Read the model definition and answer for the solid it produces. Units are mm, in the model's axes. A direction names the side the tool comes from. Give positions to 0.01 mm unless a question says otherwise; leave off trailing zeros. Write each loop counter-clockwise with the first axis right and the second up, starting at its lowest first coordinate (ties: lowest second). Pieces come first, ordered by that corner, then holes. Notation, with made-up numbers: (0, 4.5) -> (30, 4.5) arc R15 ccw to (30, 17.5) -> close; hole circle Ø3 at (-2.75, 79.25). An arc over 180 degrees is marked (long way). Use a Markdown table: item, result.
from build123d import *

# Parameters (mm, degrees)
SKETCH1_R           = 7.75
SKETCH1_W           = 44
SKETCH1_H           = 24
BOSS_EXTRUDE1_DEPTH = 65
SKETCH5_W           = 65
SKETCH5_H           = 15
SKETCH5_R           = 4.05
BOSS_EXTRUDE4_DEPTH = 83
CHAMFER1_SIZE       = 10
SKETCH6_R           = 2.75
CUT_EXTRUDE1_DEPTH  = 15
SKETCH8_R           = 2.75
BOSS_EXTRUDE5_DEPTH = 3
EXTRUDE_THIN2_DEPTH = 20
CHAMFER2_SIZE       = 5
CHAMFER3_SIZE       = 5


with BuildPart() as part:
    # Sketch1 → Boss-Extrude1 (new body)
    with BuildSketch(Plane.XY):
        Polygon((31.75, 17), (-31.75, 17), (-41.5, 17), (-41.5, -17), (-31.75, -17), (31.75, -17), (41.5, -17), (41.5, 17), align=None)
        with Locations((-31.75, 0)):
            Circle(SKETCH1_R, mode=Mode.SUBTRACT)
        with Locations((31.75, 0)):
            Circle(SKETCH1_R, mode=Mode.SUBTRACT)
        Rectangle(SKETCH1_W, SKETCH1_H, mode=Mode.SUBTRACT)
    extrude(amount=BOSS_EXTRUDE1_DEPTH)

    # Sketch5 → Boss-Extrude4 (add)
    with BuildSketch(Plane(origin=(41.5, 0, 0), x_dir=(0, 0, -1), z_dir=(1, 0, 0))):
        with Locations((-32.5, -24.5)):
            Rectangle(SKETCH5_W, SKETCH5_H)
        with Locations((-55, -24.5)):
            Circle(SKETCH5_R, mode=Mode.SUBTRACT)
        with Locations((-10, -24.5)):
            Circle(SKETCH5_R, mode=Mode.SUBTRACT)
    extrude(amount=-BOSS_EXTRUDE4_DEPTH)

    # Chamfer1
    chamfer1_edges = [part.edges().sort_by_distance(p)[0] for p in [
        (41.5, 17, 32.5),
    ]]
    chamfer(chamfer1_edges, length=CHAMFER1_SIZE)

    # Sketch6 → Cut-Extrude1 (cut)
    with BuildSketch(Plane(origin=(0, 12, 0), x_dir=(-1, 0, 0), z_dir=(0, -1, 0))):
        with Locations(Location((12, -32.5, 0), (0, 0, 90))):
            Circle(SKETCH6_R)
    extrude(amount=-CUT_EXTRUDE1_DEPTH, mode=Mode.SUBTRACT)



with BuildPart() as body_2:
    # Sketch8 → Boss-Extrude5 (new body)
    with BuildSketch(Plane(origin=(0, 37, 0), x_dir=(1, 0, 0), z_dir=(0, 1, 0))):
        Polygon((-41.5, -10), (-21, -32.5), (-41.5, -55), (-41.5, -65), (-31.5, -65), (-12, -41.5), (21.5, -65), (31.5, -65), (31.5, -55), (-3, -32.5), (31.5, -10), (31.5, 0), (21.5, 0), (-12, -21.847826087), (-31.5, 0), (-41.5, 0), align=None)
        with Locations(Location((-12, -32.5, 0), (0, 0, 90))):
            Circle(SKETCH8_R, mode=Mode.SUBTRACT)
    extrude(amount=BOSS_EXTRUDE5_DEPTH)


with BuildPart() as part_1:
    add(part.part)

    add(body_2.part)  # Extrude-Thin2 merges body 2
    # Sketch9 → Extrude-Thin2 (add)
    with BuildSketch(Plane(origin=(0, 37, 0), x_dir=(-1, 0, 0), z_dir=(0, -1, 0))):
        Polygon((41.5, -10), (41.5, 0), (31.5, 0), (31.5, -3), (38.5, -3), (38.5, -10), align=None)
        Polygon((-21.5, 0), (-31.5, 0), (-31.5, -10), (-28.5, -10), (-28.5, -3), (-21.5, -3), align=None)
    extrude_thin2 = extrude(amount=EXTRUDE_THIN2_DEPTH)

    # Mirror1: Extrude-Thin2 across plane
    add(extrude_thin2.mirror(Plane.XY.offset(32.5)))

    # Chamfer2
    chamfer2_edges = [part_1.edges().sort_by_distance(p)[0] for p in [
        (25, 37, 3),
        (28.5, 37, 6.5),
        (-38.5, 37, 58.5),
        (-35, 37, 62),
        (25, 37, 62),
        (28.5, 37, 58.5),
        (-38.5, 37, 6.5),
        (-35, 37, 3),
    ]]
    chamfer(chamfer2_edges, length=CHAMFER2_SIZE)

    # Chamfer3
    # the kernel refuses this chamfer: 5 mm, written as the material it takes off along each edge
    with BuildSketch(Plane(origin=(-41.5, 40, 42.14158506), x_dir=(0.9996219169112968, 0.0274958766105877, 0), z_dir=(0, 0, 1)), Plane(origin=(-54.35841494, 40, 65), x_dir=(0, 0.027495876610586317, -0.9996219169112968), z_dir=(1, 0, 0)), Plane(origin=(8.64158506, 40, 65), x_dir=(0, 0.027495876610586317, -0.9996219169112968), z_dir=(1, 0, 0)), Plane(origin=(31.5, 40, 77.85841494), x_dir=(-0.9996219169112968, 0.027495876610584936, 0), z_dir=(0, 0, -1)), Plane(origin=(44.35841494, 40, 0), x_dir=(0, 0.027495876610586317, 0.9996219169112968), z_dir=(-1, 0, 0)), Plane(origin=(-18.64158506, 40, 0), x_dir=(-1.1764219776297879e-15, 0.027495876610586317, 0.9996219169112968), z_dir=(-1, 0, 0)), Plane(origin=(-41.5, 40, -12.85841494), x_dir=(0.9996219169112968, 0.0274958766105877, 1.4205481831358163e-15), z_dir=(0, 0, 1))) as chamfer3_piece_1:
        Polygon((CHAMFER3_SIZE * 0.999621916911, -CHAMFER3_SIZE * 0.0274958766106), (-CHAMFER3_SIZE * 0.0274958766106, -CHAMFER3_SIZE * 0.999621916911), (0, 0), align=None)
    extrude(amount=35.71682988, mode=Mode.SUBTRACT)
    with BuildSketch(Plane(origin=(31.5, 40, 22.85841494), x_dir=(0.02749587661058701, -0.9996219169112968, 0), z_dir=(0, 0, -1))) as chamfer3_piece_2:
        Polygon((CHAMFER3_SIZE * 0.999621916911, CHAMFER3_SIZE * 0.0274958766106), (-CHAMFER3_SIZE * 0.0274958766106, CHAMFER3_SIZE * 0.999621916911), (0, 0), align=None)
    extrude(amount=35.71682988, mode=Mode.SUBTRACT)


solid = part_1.part
Item 1: A cutting plane is placed at D-D (x = -18). Give the vertices of the cut face in (y, z).
Return value:
| item | result |
|---|---|
| outline | (-32, 0) -> (-12, 0) -> (-12, 65) -> (-32, 65) -> close; (12, 0) -> (17, 0) -> (17, 65) -> (12, 65) -> close; (37, 15.13) -> (40, 15.13) -> (40, 48.73) -> (37, 48.73) -> close; hole circle Ø8.1 at (-24.5, 10); hole circle Ø8.1 at (-24.5, 55) |
Item 2: This flat-tipped pin is pushed along its axis until it touches: P1, Ø5, axis at y = 28.5, z = 6.5, coming from the +X side. Where does it stop, or does it pass through?
Return value:
| item | result |
|---|---|
| P1 | x = 31.5 |
Item 3: A cutting plane is placed at A-A (y = -10). Give the vertices of the cut face in (x, z).
Return value:
| item | result |
|---|---|
| outline | (-41.5, 0) -> (-22, 0) -> (-22, 65) -> (-41.5, 65) -> close; (22, 0) -> (41.5, 0) -> (41.5, 65) -> (22, 65) -> close |
Item 4: For a pull along Z with two mould halves and no side action, classify faces 1 (the face through (29, 29, 55)), 2 (the face through (31.5, 26, 60)), 3 (the face through (-39, 29, 55)) as +Z half, -Z half, draft (parallel to the pull), parting line (faces both ways), or undercut.
Return value:
| item | result |
|---|---|
| face 1 | undercut |
| face 2 | draft |
| face 3 | undercut |
Item 5: A tool of negligible diameter and unlimited length cuts with its end or side. For faces 4 (the face through (28.5, 25, 7)), 5 (the face through (-30.12, 38.48, 42.51)), 6 (the face through (22, 0, 32)), 7 (the face through (29, 29, 10)), from which of +Z, -Z, +X, -X, +Y, -Y can it reach the whole face along a straight path? Write none if from no direction.
Return value:
| item | result |
|---|---|
| face 4 | none |
| face 5 | -X, +Y |
| face 6 | +Z, -Z |
| face 7 | +X, -X |
Item 6: A cutting plane is placed at B-B (x = 35). Give the vertices of the cut face in (y, z).
Return value:
| item | result |
|---|---|
| outline | (-32, 0) -> (-7.04, 0) -> (-7.04, 65) -> (-32, 65) -> close; (7.04, 0) -> (13.5, 0) -> (13.5, 65) -> (7.04, 65) -> close; hole circle Ø8.1 at (-24.5, 10); hole circle Ø8.1 at (-24.5, 55) |
Item 7: Straight lines are drawn through the part: line 1 along Y through (x, z) = (-4, 42); line 2 along Y through (x, z) = (6.5, 10); line 3 along X through (y, z) = (28, 58). For each, find the intervals that lie inside material, in ascending order. Write a range as [from, to].
Return value:
| item | result |
|---|---|
| line 1 | [-32, -12], [12, 17], [37, 40] |
| line 2 | [-32, -28.55], [-20.45, -12], [12, 17], [37, 40] |
| line 3 | [-41.5, -38.5], [28.5, 31.5] |
Item 8: A cutting plane is placed at C-C (y = 21). Give the vertices of the cut face in (x, z), then the cut area to 3 significant figures.
Return value:
| item | result |
|---|---|
| outline | (-41.5, 0) -> (-31.5, 0) -> (-31.5, 3) -> (-38.5, 3) -> (-38.5, 10) -> (-41.5, 10) -> close; (-41.5, 55) -> (-38.5, 55) -> (-38.5, 62) -> (-31.5, 62) -> (-31.5, 65) -> (-41.5, 65) -> close; (21.5, 0) -> (31.5, 0) -> (31.5, 10) -> (28.5, 10) -> (28.5, 3) -> (21.5, 3) -> close; (21.5, 62) -> (28.5, 62) -> (28.5, 55) -> (31.5, 55) -> (31.5, 65) -> (21.5, 65) -> close |
| area | 204 mm^2 |
